Design review of the part built by this model. Coordinates are the model's own, in mm. Face numbers are marked on the shaded views. A direction names the side the tool comes from. Give positions to 0.01 mm unless a question says otherwise; leave off trailing zeros. Write each loop counter-clockwise with the first axis right and the second up, starting at its lowest first coordinate (ties: lowest second). Pieces come first, ordered by that corner, then holes. Notation, with made-up numbers: M 73,-37.5 L 94,-37.5 A21 cw 94,-2.5 Z; hole C 10,-12.75 d1. An arc over 180 degrees is marked long. Answer in a Markdown table with one row per item.
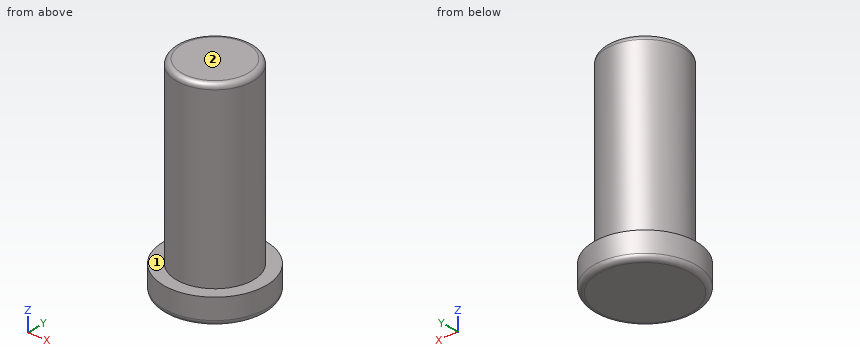
```python
from build123d import *

# Parameters (mm, degrees)
F0_R     = 10
F1_DEPTH = 5
F2_R     = 7.5
F3_DEPTH = 35
F4_R     = 1
F5_R     = 1


with BuildPart() as f1:
    # F0 (on Top) → F1 (new body)
    with BuildSketch(Plane.XY):
        Circle(F0_R)
    extrude(amount=F1_DEPTH)

    # F2 (on face) → F3 (join)
    with BuildSketch(Plane.XY.offset(5)):
        Circle(F2_R)
    extrude(amount=F3_DEPTH)

    # F4
    f4_edges = [f1.edges().sort_by_distance(p)[0] for p in [
        (-7.5, 0, 40),
    ]]
    fillet(f4_edges, radius=F4_R)

    # F5
    f5_edges = [f1.edges().sort_by_distance(p)[0] for p in [
        (-10, 0, 0),
    ]]
    fillet(f5_edges, radius=F5_R)


solid = f1.part
```
1) Add section A-A (y = 0). Write out the cut boundary in (x, z), and give its area (3 significant figures).
Geometry says:
| item | result |
|---|---|
| outline | M -10,1 A1 ccw -9,0 L 9,0 A1 ccw 10,1 L 10,5 L 7.5,5 L 7.5,39 A1 ccw 6.5,40 L -6.5,40 A1 ccw -7.5,39 L -7.5,5 L -10,5 Z |
| area | 624 mm^2 |
2) Add section C-C (z = 13.5). Write out the cut boundary in (x, y), and give its area (3 significant figures).
Geometry says:
| item | result |
|---|---|
| outline | C 0,0 d15 |
| area | 177 mm^2 |
3) Insertion check: P1, Ø6, axis at x = -6.5, z = 16.5, coming from the -Y side; P2, Ø10, axis at x = 7.5, z = 17.5, coming from the -Y side; P3, Ø1.5, axis at x = 6.5, z = 18.5, coming from the -Y side. Each pin has a flat end and moves straight along its axis. Give the tip position at first contact, or say it passes through.
Geometry says:
| item | result |
|---|---|
| P1 | y = -6.63 |
| P2 | y = -7.07 |
| P3 | y = -4.82 |
4) To check wall thickness, follow probe 1 along X at (y, z) = (3.75, 12.5); probe 2 along X at (y, z) = (0.25, 7.5); probe 3 along Z at (x, y) = (-1.75, -8.25). State the ranges of each line that lie inside material, in increasing order. Write a range as [from, to].
Geometry says:
| item | result |
|---|---|
| probe 1 | [-6.5, 6.5] |
| probe 2 | [-7.5, 7.5] |
| probe 3 | [0, 5] |
5) Add section D-D (z = 4). Write out the cut boundary in (x, y), and give its area (3 significant figures).
Geometry says:
| item | result |
|---|---|
| outline | C 0,0 d20 |
| area | 314 mm^2 |
6) For the marked faces 1 and 2, list the 3-axis set-ups (+Z, -Z, +X, -X, +Y, -Y) from which the entire face can be reached by the end or side of a thin tool; tool diameter is ignored.
Geometry says:
| item | result |
|---|---|
| face 1 | +Z |
| face 2 | +Z, +X, -X, +Y, -Y |
